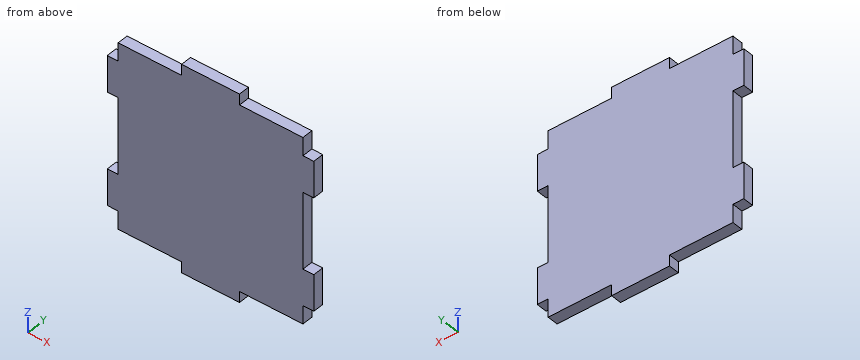
Autodesk Inventor part; units mm, degrees
ref_plane "YZ Plane" through (0, 0, 0) normal (1, 0, 0) x (0, 1, 0)
ref_plane "XZ Plane" through (0, 0, 0) normal (0, 1, 0) x (-1, 0, 0)
ref_plane "XY Plane" through (0, 0, 0) normal (0, 0, 1) x (1, 0, 0)
sketch "Sketch1" plane through (0, 0, 0) normal (0, 1, 0) x (-1, 0, 0)
  line L0 (-28.5, -57) -> (-28.5, -28.5) construction
  line L1 (-28.5, -28.5) -> (-57, -28.5) construction
  line L2 (0, -49) -> (-3, -49)
  line L3 (-3, -49) -> (-3, -57)
  line L4 (0, -49) -> (0, -39)
  line L5 (0, -39) -> (-3, -39)
  line L6 (-3, -39) -> (-3, -28.5)
  line L7 (0, -8) -> (-3, -8)
  line L8 (-3, -8) -> (-3, 0)
  line L9 (0, -18) -> (-3, -18)
  line L10 (-3, -18) -> (-3, -28.5)
  line L11 (0, -8) -> (0, -18)
  line L12 (0, -39) -> (0, -49)
  line L13 (0, -49) -> (0, -39)
  line L14 (0, -18) -> (0, -8)
  line L15 (-57, -49) -> (-54, -49)
  line L16 (-54, -49) -> (-54, -57)
  line L17 (-57, -49) -> (-57, -39)
  line L18 (-57, -39) -> (-54, -39)
  line L19 (-54, -39) -> (-54, -28.5)
  line L20 (-57, -8) -> (-54, -8)
  line L21 (-54, -8) -> (-54, 0)
  line L22 (-57, -18) -> (-54, -18)
  line L23 (-54, -18) -> (-54, -28.5)
  line L24 (-57, -8) -> (-57, -18)
  line L25 (-57, -39) -> (-57, -49)
  line L26 (-57, -49) -> (-57, -39)
  line L27 (-57, -18) -> (-57, -8)
  line L28 (-57, -49) -> (-57, -39)
  line L29 (-57, -18) -> (-57, -8)
  line L30 (-28.5, -54) -> (-36.5, -54)
  line L31 (-36.5, -54) -> (-36.5, -57)
  line L32 (-28.5, -54) -> (-20.5, -54)
  line L33 (-20.5, -54) -> (-20.5, -57)
  line L34 (-3, -57) -> (-20.5, -57)
  line L35 (-36.5, -57) -> (-54, -57)
  line L36 (-28.5, -3) -> (-36.5, -3)
  line L37 (-36.5, -3) -> (-36.5, 0)
  line L38 (-20.5, -3) -> (-20.5, 0)
  line L39 (-28.5, -3) -> (-20.5, -3)
  line L40 (-54, 0) -> (-36.5, 0)
  line L41 (-20.5, 0) -> (-3, 0)
  point P0 (0, 0)
  point P1 (0, -57)
  dimension "d3" = 3
  dimension "d4" = 10
  dimension "d5" = 3
  dimension "d6" = 3
  dimension "d7" = 8
extrude "Extrusion1" add sketch "Sketch1" along normal blind 3
sketch "Sketch2" plane through (0, 3, 0) normal (0, 1, 0) x (1, 0, 0)
  line L0 (36.5, 0) -> (54, 0)
  line L1 (36.5, 3) -> (36.5, 0)
  line L2 (36.5, 0) -> (36.5, 3)
  line L3 (36.5, 3) -> (54, 3)
  line L4 (54, 0) -> (54, 8)
  line L5 (20.5, 0) -> (20.5, 3)
  line L6 (20.5, 0) -> (20.5, 3)
  line L7 (20.5, 3) -> (36.5, 3)
  line L8 (20.5, 3) -> (36.5, 3)
  line L9 (36.5, 3) -> (36.5, 0)
  line L10 (3, 0) -> (20.5, 0)
  line L11 (20.5, 0) -> (20.5, 3)
  line L12 (3, 0) -> (3, 3)
  line L13 (3, 8) -> (3, 0)
  line L14 (20.5, 3) -> (3, 3)
  point P0 (0, 0)
extrude "Extrusion2" cut sketch "Sketch2" against normal up to surface (3 mm away)
sketch "Sketch3" plane through (0, 3, 0) normal (0, 1, 0) x (1, 0, 0)
  line L0 (3, 3) -> (20.5, 3)
  line L1 (3, 3) -> (54, 3)
  line L2 (20.5, 3) -> (20.5, 0)
  line L3 (36.5, 54) -> (20.5, 54)
  line L4 (28.5, 54) -> (28.5, 14.4088) construction
  line L5 (54, 3) -> (36.5, 3)
  line L6 (36.5, 3) -> (36.5, 0)
  line L7 (20.5, 0) -> (36.5, 0)
  point P0 (0, 0)
  dimension "d12" = 17.5
extrude "Extrusion3" add sketch "Sketch3" against normal up to surface (3 mm away)
sketch "Sketch4" plane through (0, 3, 0) normal (0, 1, 0) x (1, 0, 0)
  line L0 (36.5, 54) -> (20.5, 54)
  line L1 (20.5, 54) -> (3, 54)
  line L2 (3, 57) -> (3, 49)
  line L3 (36.5, 57) -> (36.5, 54)
  line L4 (36.5, 54) -> (54, 54)
  line L5 (54, 49) -> (54, 57)
  line L6 (20.5, 57) -> (3, 57)
  line L7 (3, 54) -> (3, 57)
  line L8 (3, 57) -> (20.5, 57)
  line L9 (20.5, 57) -> (20.5, 54)
  line L10 (36.5, 57) -> (36.5, 54)
  line L11 (54, 57) -> (36.5, 57)
  line L12 (36.5, 57) -> (54, 57)
  line L13 (54, 57) -> (54, 54)
  point P0 (0, 0)
extrude "Extrusion4" cut sketch "Sketch4" against normal up to surface (3 mm away)
sketch "Sketch5" plane through (0, 3, 0) normal (0, 1, 0) x (1, 0, 0)
  line L0 (54, 18) -> (54, 39)
  line L1 (54, 28.5) -> (3, 28.5) construction
  line L2 (3, 39) -> (3, 18)
  line L3 (3, 3) -> (20.5, 3)
  line L4 (3, 3) -> (20.5, 3)
  line L5 (20.5, 3) -> (20.5, 0)
  line L6 (20.5, 0) -> (36.5, 0)
  line L7 (20.5, 0) -> (36.5, 0)
  line L8 (36.5, 0) -> (36.5, 3)
  line L9 (36.5, 3) -> (54, 3)
  line L10 (36.5, 3) -> (54, 3)
  line L11 (3, 54) -> (20.5, 54)
  line L12 (20.5, 54) -> (20.5, 57)
  line L13 (20.5, 57) -> (36.5, 57)
  line L14 (36.5, 57) -> (36.5, 54)
  line L15 (36.5, 54) -> (54, 54)
  line L16 (20.5, 54) -> (36.5, 54)
  line L17 (54, 54) -> (3, 54)
  point P0 (0, 0)
extrude "Extrusion5" add sketch "Sketch5" against normal up to surface (3 mm away)
properties part number "Inferior" material "LCP Plastic"
Geometry: final body of the model. Coordinates: model frame, mm. Round coordinates to 2 decimals unless told otherwise and drop trailing zeros. Order: outer loops, then holes, each group sorted by start corner. A loop starts at its lowest first (then second) coordinate and runs counter-clockwise, first axis right, second up. Notation, with made-up numbers: (12.25, -2) - (62.25, -2) arc R24 cw to (62.25, 35) - close; hole circle Ø1 at (41.25, 71). An arc over 180 degrees is marked (long way). Write item = value, one per line. Start each with the question number.
Q1. Cut plane A-A on y = 1.5. Return the cut outline in (x, z), and give its area (3 significant figures).
Q2. Cut plane B-B on z = -6. Return the cut outline in (x, y), and give its area (3 significant figures).
Q3. Ray query, line 1 (X direction, y = 2.95, z = -37.5); line 2 (Z direction, x = 37, y = 2.2). Return the intervals inside material, ascending. Write a range as from..to.
Q4. Cut plane C-C on x = 43.5. Return the cut outline in (y, z).
Q5. Pin query (flat end, axial travel): pin 1 (0.9 mm diameter, centred on x = 1, y = 1.5, fed in from -Z); pin 2 (1.5 mm diameter, centred on y = 1.5, z = -51.5, fed in from -X); pin 3 (0.9 mm diameter, centred on y = 1.5, z = -6.5, fed in from +X). Return the tip coordinate at first contact, or that it passes through.
Outcome:
q1.outline = (0, -49) - (3, -49) - (3, -54) - (20.5, -54) - (20.5, -57) - (36.5, -57) - (36.5, -54) - (54, -54) - (54, -49) - (57, -49) - (57, -39) - (54, -39) - (54, -18) - (57, -18) - (57, -8) - (54, -8) - (54, -3) - (36.5, -3) - (36.5, 0) - (20.5, 0) - (20.5, -3) - (3, -3) - (3, -8) - (0, -8) - (0, -18) - (3, -18) - (3, -39) - (0, -39) - close
q1.area = 2,820 mm^2
q2.outline = (3, 0) - (54, 0) - (54, 3) - (3, 3) - close
q2.area = 153 mm^2
q3.line_1 = 3..54
q3.line_2 = -54..-3
q4.outline = (0, -54) - (3, -54) - (3, -3) - (0, -3) - close
q5.pin_1 = -49
q5.pin_2 = 3
q5.pin_3 = 54
